```python
from build123d import *

# Parameters (mm, degrees)
SKETCH1_R           = 8.7503
SKETCH1_R_2         = 3.175
BOSS_EXTRUDE1_DEPTH = 5.08
SKETCH2_R           = 10.2235
SKETCH2_R_2         = 3.175
BOSS_EXTRUDE2_DEPTH = 1.143
SKETCH3_R           = 6.604
BOSS_EXTRUDE3_DEPTH = 11.43
SKETCH4_R           = 3.175
CUT_EXTRUDE1_DEPTH  = 12.43


with BuildPart() as part:
    # Sketch1 → Boss-Extrude1 (new body)
    with BuildSketch(Plane(origin=(0, 0, 0), x_dir=(1, 0, 0), z_dir=(0, 1, 0))):
        Circle(SKETCH1_R)
        Circle(SKETCH1_R_2, mode=Mode.SUBTRACT)
    extrude(amount=BOSS_EXTRUDE1_DEPTH)

    # Sketch2 → Boss-Extrude2 (add)
    with BuildSketch(Plane(origin=(0, 5.08, 0), x_dir=(1, 0, 0), z_dir=(0, 1, 0))):
        Circle(SKETCH2_R)
        Circle(SKETCH2_R_2, mode=Mode.SUBTRACT)
    extrude(amount=BOSS_EXTRUDE2_DEPTH)

    # Sketch3 → Boss-Extrude3 (add)
    with BuildSketch(Plane(origin=(0, 6.223, 0), x_dir=(1, 0, 0), z_dir=(0, 1, 0))):
        Circle(SKETCH3_R)
    extrude(amount=BOSS_EXTRUDE3_DEPTH)

    # Sketch4 → Cut-Extrude1 (cut, through all)
    with BuildSketch(Plane.XZ.offset(-6.223)):
        Circle(SKETCH4_R)
    extrude(amount=-CUT_EXTRUDE1_DEPTH, mode=Mode.SUBTRACT)


solid = part.part
```
Source: CAD feature listing. Evaluate the final solid. Frame: model axes, mm. A direction names the side the tool comes from. Round coordinates to 2 decimals unless told otherwise and drop trailing zeros. Loops run counter-clockwise (first coordinate to the right, second up) from the corner with the lowest first, then second, coordinate; pieces in that order, holes last.
(1) Material intervals for probe 1 along Z at (x, y) = (0, 9.5) (3 decimals); probe 2 along Z at (x, y) = (0, 4.5) (3 decimals), sorted ascending.
From the geometry:
probe 1: z = -6.604 to -3.175, 3.175 to 6.604
probe 2: z = -8.75 to -3.175, 3.175 to 8.75
(2) Contact query for flat-ended pins moving along their axis: pin 1 Ø10 at (x, z) = (1.5, 8) entering from +Y; pin 2 Ø4 at (y, z) = (2.5, -2) entering from +X; pin 3 Ø8 at (x, y) = (2.5, 11) entering from -Z; pin 4 Ø2 at (x, z) = (-7, 8) entering from +Y. Output: stop coordinate, or through.
From the geometry:
pin 1: stops at y = 17.65
pin 2: stops at x = 8.75
pin 3: stops at z = -6.6
pin 4: stops at y = 6.22
(3) Access query for faces 1 (the flat face through (0, 6.223, 7)), 2 (the flat face through (8, 5.08, -5)), 3 (the flat face through (4, 0, 0)). Directions: +Z, -Z, +X, -X, +Y, -Y. A direction counts if a zero-diameter tool reaches every point of the face in a straight line with its end or side. Return the directions, or none.
From the geometry:
face 1: +Y
face 2: -Y
face 3: +Z, -Z, +X, -X, -Y
(4) Section query B-B (z = 0). Output: boundary loops of the cut face in (x, y) (1 decimal), and give its area (3 significant figures).
From the geometry:
outline: (-10.2, 5.1) - (-8.8, 5.1) - (-8.8, 0) - (-3.2, 0) - (-3.2, 17.7) - (-6.6, 17.7) - (-6.6, 6.2) - (-10.2, 6.2) - close; (3.2, 0) - (8.8, 0) - (8.8, 5.1) - (10.2, 5.1) - (10.2, 6.2) - (6.6, 6.2) - (6.6, 17.7) - (3.2, 17.7) - close
area: 151 mm2
(5) Section query D-D (x = -5.5). Output: boundary loops of the cut face in (y, z), and give its area (3 significant figures).
From the geometry:
outline: (0, -6.81) - (5.08, -6.81) - (5.08, -8.62) - (6.22, -8.62) - (6.22, -3.66) - (17.65, -3.66) - (17.65, 3.66) - (6.22, 3.66) - (6.22, 8.62) - (5.08, 8.62) - (5.08, 6.81) - (0, 6.81) - close
area: 172 mm2
(6) Section query C-C (y = 14.25). Output: boundary loops of the cut face in (x, z) (3 decimals), and give its area (3 significant figures).
From the geometry:
outline: circle Ø13.208 at (0, 0); hole circle Ø6.35 at (0, 0)
area: 105 mm2
(7) Section query A-A (x = 0). Output: boundary loops of the cut face in (y, z) (1 decimal).
From the geometry:
outline: (0, -8.8) - (5.1, -8.8) - (5.1, -10.2) - (6.2, -10.2) - (6.2, -6.6) - (17.7, -6.6) - (17.7, -3.2) - (0, -3.2) - close; (0, 3.2) - (17.7, 3.2) - (17.7, 6.6) - (6.2, 6.6) - (6.2, 10.2) - (5.1, 10.2) - (5.1, 8.8) - (0, 8.8) - close
